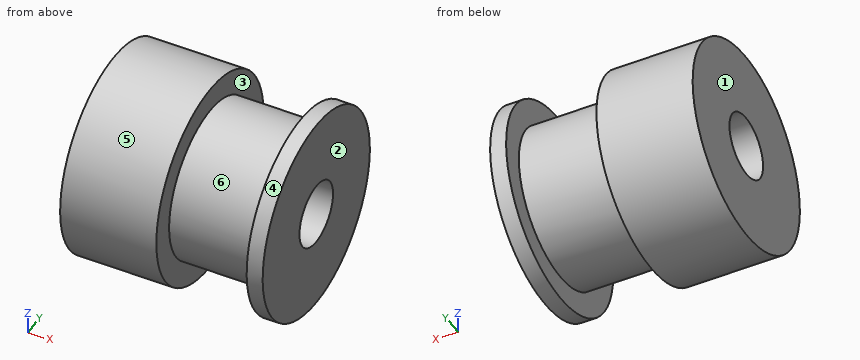
from build123d import *

# Parameters (mm, degrees)
SKETCH1_R           = 7.975
BOSS_EXTRUDE1_DEPTH = 15.83
SKETCH2_W           = 7.06
SKETCH2_H           = 1.895
SKETCH3_R           = 2.5
CUT_EXTRUDE1_DEPTH  = 16.83


with BuildPart() as part:
    # Sketch1 → Boss-Extrude1 (new body)
    with BuildSketch(Plane(origin=(0, 0, 0), x_dir=(0, 0, -1), z_dir=(1, 0, 0))):
        Circle(SKETCH1_R)
    extrude(amount=BOSS_EXTRUDE1_DEPTH)

    # Sketch2 → Cut-Revolve1 (revolve, cut)
    with BuildSketch(Plane.XY):
        with Locations((11.05, 7.0275)):
            Rectangle(SKETCH2_W, SKETCH2_H)
    revolve(axis=Axis((0, 0, 0), (1, 0, 0)), mode=Mode.SUBTRACT)

    # Sketch3 → Cut-Extrude1 (cut, through all)
    with BuildSketch(Plane(origin=(15.83, 0, 0), x_dir=(0, 0, -1), z_dir=(1, 0, 0))):
        Circle(SKETCH3_R)
    extrude(amount=-CUT_EXTRUDE1_DEPTH, mode=Mode.SUBTRACT)


solid = part.part
Design review of the part built by this model. Coordinates are the model's own, in mm. Face numbers are marked on the shaded views. A direction names the side the tool comes from. Round coordinates to 2 decimals unless told otherwise and drop trailing zeros. Write each loop counter-clockwise with the first axis right and the second up, starting at its lowest first coordinate (ties: lowest second). Pieces come first, ordered by that corner, then holes. Notation, with made-up numbers: (-2, 48) -> (7, 48) arc R34 ccw to (7, 84) -> close; hole circle Ø9 at (-11.75, 15). An arc over 180 degrees is marked (long way). One line per item, written item: value. Start each with the question number.
Q1. Add section D-D (z = 3.5). Give the boundary of the cut face in (x, y).
Q2. Add section B-B (y = -1.25). Give the boundary of the cut face in (x, z).
Q3. The part is to be moulded in two halves that separate along X. For the marked faces 1, 2, 3 and 4, say which applies: pulls with the +X half, pulls with the -X half, needs draft (parallel to the pull), parting line crosses it, or undercut.
Q4. Add section A-A (z = 0). Give the boundary of the cut face in (x, y) (3 decimals).
Q5. Insertion check: P1, Ø8, axis at x = 4, z = -5.5, coming from the +Y side; P2, Ø1, axis at x = 6, y = -2, coming from the -Z side; P3, Ø4, axis at x = 11, z = 5.5, coming from the +Y side. Each pin has a flat end and moves straight along its axis. Give the tip position at first contact, or say it passes through.
Q6. To check wall thickness, follow probe 1 along X at (y, z) = (4.5, -5.25); probe 2 along Y at (x, z) = (6, 0) (3 decimals); probe 3 along Y at (x, z) = (9, -1.25). State the ranges of each line that lie inside material, in increasing order.
Q7. Add section C-C (x = 4.25). Give the boundary of the cut face in (y, z) (3 decimals), then the cut area to 3 significant figures.
Q8. Tool access review of the marked faces 5 and 6: name each direction out of +Z, -Z, +X, -X, +Y, -Y from which nothing blocks a thin tool from reaching the whole face with its end or side.
Response:
1. outline: (0, -7.17) -> (7.52, -7.17) -> (7.52, -4.97) -> (14.58, -4.97) -> (14.58, -7.17) -> (15.83, -7.17) -> (15.83, 7.17) -> (14.58, 7.17) -> (14.58, 4.97) -> (7.52, 4.97) -> (7.52, 7.17) -> (0, 7.17) -> close
2. outline: (0, -7.88) -> (7.52, -7.88) -> (7.52, -5.95) -> (14.58, -5.95) -> (14.58, -7.88) -> (15.83, -7.88) -> (15.83, -2.17) -> (0, -2.17) -> close; (0, 2.17) -> (15.83, 2.17) -> (15.83, 7.88) -> (14.58, 7.88) -> (14.58, 5.95) -> (7.52, 5.95) -> (7.52, 7.88) -> (0, 7.88) -> close
3. face 1: pulls with the -X half
3. face 2: pulls with the +X half
3. face 3: undercut
3. face 4: needs draft
4. outline: (0, -7.975) -> (7.52, -7.975) -> (7.52, -6.08) -> (14.58, -6.08) -> (14.58, -7.975) -> (15.83, -7.975) -> (15.83, -2.5) -> (0, -2.5) -> close; (0, 2.5) -> (15.83, 2.5) -> (15.83, 7.975) -> (14.58, 7.975) -> (14.58, 6.08) -> (7.52, 6.08) -> (7.52, 7.975) -> (0, 7.975) -> close
5. P1: stops at y = 7.83
5. P2: stops at z = -7.83
5. P3: stops at y = 4.97
6. probe 1: x = 0 to 7.52, 14.58 to 15.83
6. probe 2: y = -7.975 to -2.5, 2.5 to 7.975
6. probe 3: y = -5.95 to -2.17, 2.17 to 5.95
7. outline: circle Ø15.95 at (0, 0); hole circle Ø5 at (0, 0)
7. area: 180 mm^2
8. face 5: +X, -X
8. face 6: none
